Geometry: final body of the model. Coordinates: model frame, mm. Face numbers are marked on the shaded views. A direction names the side the tool comes from. Coordinates: 2 decimals unless noted, no trailing zeros. Loops run counter-clockwise (first coordinate to the right, second up) from the corner with the lowest first, then second, coordinate; pieces in that order, holes last. Notation, with made-up numbers: (-11.5, 78) - (20.5, 78) arc R18 cw to (20.5, 101) - close; hole circle Ø9 at (69.5, 11). An arc over 180 degrees is marked (long way). Return JSON: item names as keys, results as strings.
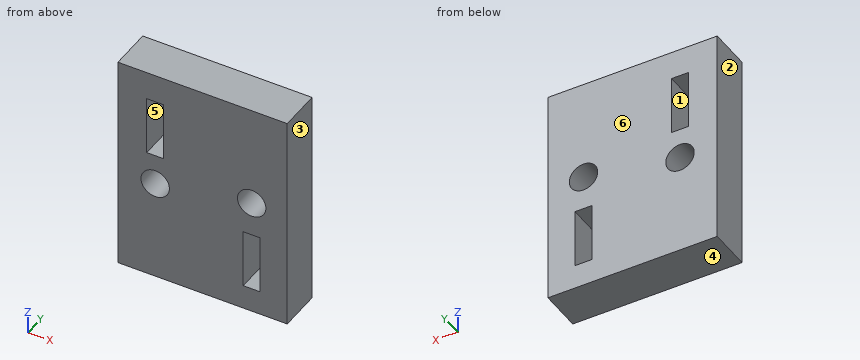
from build123d import *

# Parameters (mm, degrees)
BOX002_W        = 20
BOX002_H        = 5
BOX002_DEPTH    = 26
SKETCH_R        = 1.68
SKETCH_W        = 2
SKETCH_H        = 7
POCKET014_DEPTH = 5


with BuildPart() as part:
    # Box002 → Box002 (new body)
    with BuildSketch(Plane(origin=(20.8, -5, 0), x_dir=(1, 0, 0), z_dir=(0, 0, 1))):
        with Locations((10, 2.5)):
            Rectangle(BOX002_W, BOX002_H)
    extrude(amount=BOX002_DEPTH)

    # Sketch → Pocket014 (cut)
    with BuildSketch(Plane(origin=(20.8, -5, 0), x_dir=(1, 0, 0), z_dir=(0, -1, 0))):
        with Locations((4.4, 12)):
            Circle(SKETCH_R)
        with Locations((15.8, 14)):
            Circle(SKETCH_R)
        with Locations((4.4, 19.125)):
            Rectangle(SKETCH_W, SKETCH_H)
        with Locations((15.8, 6.4)):
            Rectangle(SKETCH_W, SKETCH_H)
    extrude(amount=-POCKET014_DEPTH, mode=Mode.SUBTRACT)


solid = part.part
Item 1: First-contact query: pin 1 Ø4 at (x, z) = (34.5, 5) entering from +Y. Flat tip, straight axial feed; report the tip coordinate or a pass-through.
Worked out:
{"pin 1": "y = 0"}
Item 2: Section query A-A, the plane z = 21. Return loops of the section in (x, y), and give its area (3 significant figures).
Worked out:
{"outline": "(20.8, -5) - (24.2, -5) - (24.2, 0) - (20.8, 0) - close; (26.2, -5) - (40.8, -5) - (40.8, 0) - (26.2, 0) - close", "area": "90.0 mm^2"}
Item 3: Section query C-C, the plane y = -2.1. Return loops of the section in (x, z) (3 decimals).
Worked out:
{"outline": "(20.8, 0) - (40.8, 0) - (40.8, 26) - (20.8, 26) - close; hole circle Ø3.36 at (25.2, 12); hole (24.2, 15.625) - (26.2, 15.625) - (26.2, 22.625) - (24.2, 22.625) - close; hole circle Ø3.36 at (36.6, 14); hole (35.6, 2.9) - (37.6, 2.9) - (37.6, 9.9) - (35.6, 9.9) - close"}
Item 4: Reachability of the marked faces 5 and 6 from +Z, -Z, +X, -X, +Y, -Y: full face, straight path, thin tool, end or side. Return the list, or none.
Worked out:
{"face 5": "+Y, -Y", "face 6": "+Z, -Z, +X, -X, +Y"}
Item 5: Ray query, probe 1 along Z at (x, y) = (25.2, -1) (3 decimals); probe 2 along Z at (x, y) = (36.6, -3.05); probe 3 along X at (y, z) = (-3.95, 5.25). Return the intervals inside material, ascending. Write a range as from..to.
Worked out:
{"probe 1": "0..10.32, 13.68..15.625, 22.625..26", "probe 2": "0..2.9, 9.9..12.32, 15.68..26", "probe 3": "20.8..35.6, 37.6..40.8"}
Item 6: Section query B-B, the plane x = 36.6. Return loops of the section in (y, z), and give its area (3 significant figures).
Worked out:
{"outline": "(-5, 0) - (0, 0) - (0, 2.9) - (-5, 2.9) - close; (-5, 9.9) - (0, 9.9) - (0, 12.32) - (-5, 12.32) - close; (-5, 15.68) - (0, 15.68) - (0, 26) - (-5, 26) - close", "area": "78.2 mm^2"}
Item 7: Section query D-D, the plane z = 14. Return loops of the section in (x, y).
Worked out:
{"outline": "(20.8, -5) - (34.92, -5) - (34.92, 0) - (20.8, 0) - close; (38.28, -5) - (40.8, -5) - (40.8, 0) - (38.28, 0) - close"}
Item 8: Mould query, pull axis X, two halves, no side actions, for the marked faces 1, 2, 3 and 4. Classes: +X half, -X half, draft (parallel to the pull), parting line (faces both ways), or undercut.
Worked out:
{"face 1": "undercut", "face 2": "-X half", "face 3": "+X half", "face 4": "draft"}
